Print and shaded views of the part. All mm, measured from the part's lowest x, y and z. Coordinates: 2 decimals unless noted, no trailing zeros. Order: outer loops, then holes, each group sorted by start corner. A loop starts at its lowest first (then second) coordinate and runs counter-clockwise, first axis right, second up. Notation, with made-up numbers: M 16.25,-30.5 L 28.25,-30.5 A24 ccw 28.25,-17.5 Z; hole C 0,70.25 d8. An arc over 180 degrees is marked long. One line per item, written item: value.
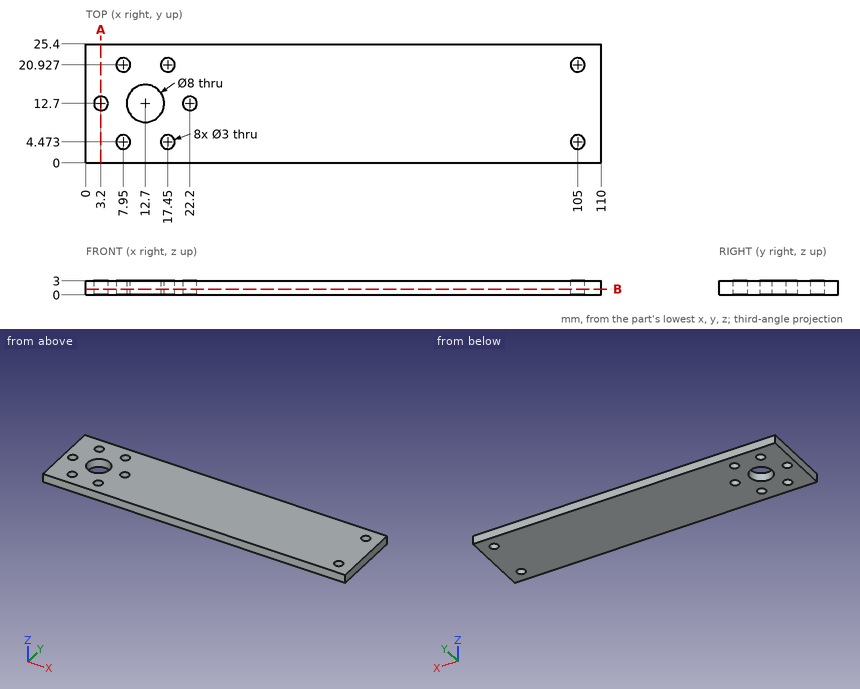
Q1. Slice it at A-A (x = 3.2). List the corners of the cut face in (y, z).
Recorded:
outline: M 0,0 L 11.2,0 L 11.2,3 L 0,3 Z; M 14.2,0 L 25.4,0 L 25.4,3 L 14.2,3 Z
Q2. Drill centre lines: line 1 along Y through (x, z) = (17.45, 1.2); line 2 along X through (y, z) = (20.75, 2.25); line 3 along X through (y, z) = (13, 2.7). Where is each one in solid material? Low to high.
Recorded:
line 1: y = 0 to 2.97, 5.97 to 19.43, 22.43 to 25.4
line 2: x = 0 to 6.46, 9.44 to 15.96, 18.94 to 103.51, 106.49 to 110
line 3: x = 0 to 1.73, 4.67 to 8.71, 16.69 to 20.73, 23.67 to 110
Q3. Pin check, flat tip, straight feed: pin 1 Ø2.5 at (x, y) = (3.2, 12.7) entering from -Z. Stop position of the tip, or through.
Recorded:
pin 1: passes through
Q4. Slice it at B-B (z = 1.25). Give the number of separate pieces and of enclosed holes in the cut face, plus the area to 3 significant figures.
Recorded:
separate pieces: 1
enclosed holes: 9
area: 2,690 mm^2
